The listing builds one solid part. Answer for the finished solid, in the listing's coordinates (mm). Face numbers are marked on the shaded views. A direction names the side the tool comes from. Coordinates: 2 decimals unless noted, no trailing zeros. Order: outer loops, then holes, each group sorted by start corner. A loop starts at its lowest first (then second) coordinate and runs counter-clockwise, first axis right, second up. Notation, with made-up numbers: (32, 79) - (45, 79) arc R16 ccw to (45, 84) - close; hole circle Ø5 at (19.5, 25). An arc over 180 degrees is marked (long way). Use a Markdown table: item, result. Add a question column.
Item 1: The mould has two halves that part along Y. Classify the marked faces 1, 2, 3 and 4: released by +Y, released by -Y, zero draft, split by the parting line, or undercut.
Item 2: The part is cut by section B-B, the plane x = 0. Give the vertices of the cut face in (y, z) (1 decimal), then the cut area to 3 significant figures.
Item 3: The part is cut by section A-A, the plane y = 0. Give the vertices of the cut face in (x, z) (3 decimals).
Item 4: Flat-ended cylindrical pins translate along their axes: P1, Ø10, axis at x = 0, y = 0, coming from the -Z side; P2, Ø5, axis at x = 17.78, y = 0, coming from the -Z side; P3, Ø2, axis at x = 8.5, z = 3, coming from the +Y side; P4, Ø5, axis at x = 2, z = 6.5, coming from the +Y side. Find the tip coordinate at first contact, or state that the pin passes through.
Item 5: The part is cut by section D-D, the plane x = -19.5. Give the vertices of the cut face in (y, z) (3 decimals).
Item 6: The part is cut by section C-C, the plane y = -20. Give the vertices of the cut face in (x, z) (3 decimals).
Item 7: Find the intervals of material crossed by line 1 along X through (y, z) = (-2, 6); line 2 along X through (y, z) = (-0.5, 7); line 3 along Y through (x, z) = (-2, 3.75), in increasing order.
Item 8: For the marked faces 5 and 6, determine the directions among +Z, -Z, +X, -X, +Y, -Y from which every point of the face is accessible in a straight line to the end or side of a thin tool.
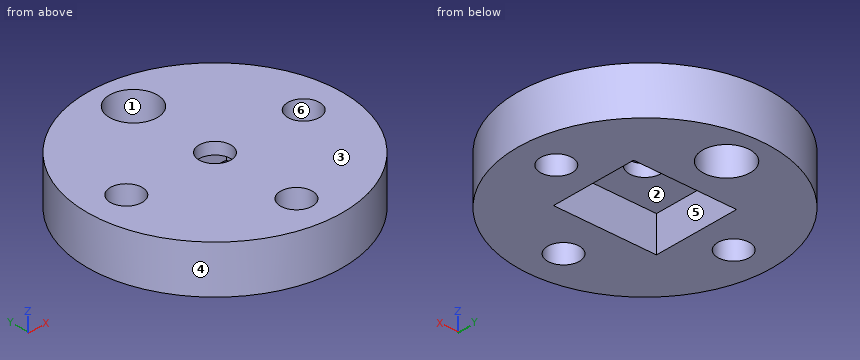
from build123d import *

# Parameters (mm, degrees)
SKETCH1_R           = 25.4
BOSS_EXTRUDE1_DEPTH = 9.525
SKETCH2_W           = 20.6375
SKETCH2_H           = 17.4625
CUT_EXTRUDE1_DEPTH  = 7.14375
SKETCH3_R           = 3.175
CUT_EXTRUDE9_DEPTH  = 15.5575
SKETCH5_R           = 4.7625
SKETCH5_R_2         = 3.175
CUT_EXTRUDE10_DEPTH = 15.5575


with BuildPart() as part:
    # Sketch1 → Boss-Extrude1 (new body)
    with BuildSketch(Plane.XY):
        with Locations(Location((0, 0, 0), (0, 0, 180))):
            Circle(SKETCH1_R)
    extrude(amount=BOSS_EXTRUDE1_DEPTH)

    # Sketch2 → Cut-Extrude1 (cut)
    with BuildSketch(Plane.XY):
        Rectangle(SKETCH2_W, SKETCH2_H)
    extrude(amount=CUT_EXTRUDE1_DEPTH, mode=Mode.SUBTRACT)

    # Sketch3 → Cut-Extrude9 (cut)
    with BuildSketch(Plane(origin=(0, 0, 7.14375), x_dir=(-1, 0, 0), z_dir=(0, 0, -1))):
        Circle(SKETCH3_R)
    extrude(amount=-CUT_EXTRUDE9_DEPTH, mode=Mode.SUBTRACT)

    # Sketch5 → Cut-Extrude10 (cut)
    with BuildSketch(Plane.XY.offset(9.525)):
        with Locations((0, 17.78)):
            Circle(SKETCH5_R)
        with Locations((17.78, 0)):
            Circle(SKETCH5_R_2)
        with Locations((0, -17.768897269)):
            Circle(SKETCH5_R_2)
        with Locations((-17.78, 0)):
            Circle(SKETCH5_R_2)
    extrude(amount=-CUT_EXTRUDE10_DEPTH, mode=Mode.SUBTRACT)


solid = part.part
Solution:
| question | item | result |
|---|---|---|
| 1 | face 1 | undercut |
| 1 | face 2 | undercut |
| 1 | face 3 | zero draft |
| 1 | face 4 | split by the parting line |
| 2 | outline | (-25.4, 0) - (-20.9, 0) - (-20.9, 9.5) - (-25.4, 9.5) - close; (-14.6, 0) - (-8.7, 0) - (-8.7, 7.1) - (-3.2, 7.1) - (-3.2, 9.5) - (-14.6, 9.5) - close; (3.2, 7.1) - (8.7, 7.1) - (8.7, 0) - (13, 0) - (13, 9.5) - (3.2, 9.5) - close; (22.5, 0) - (25.4, 0) - (25.4, 9.5) - (22.5, 9.5) - close |
| 2 | area | 193 mm2 |
| 3 | outline | (-25.4, 0) - (-20.955, 0) - (-20.955, 9.525) - (-25.4, 9.525) - close; (-14.605, 0) - (-10.319, 0) - (-10.319, 7.144) - (-3.175, 7.144) - (-3.175, 9.525) - (-14.605, 9.525) - close; (3.175, 7.144) - (10.319, 7.144) - (10.319, 0) - (14.605, 0) - (14.605, 9.525) - (3.175, 9.525) - close; (20.955, 0) - (25.4, 0) - (25.4, 9.525) - (20.955, 9.525) - close |
| 4 | P1 | stops at z = 7.14 |
| 4 | P2 | passes through |
| 4 | P3 | stops at y = 24.27 |
| 4 | P4 | stops at y = 25.4 |
| 5 | outline | (-16.276, 0) - (-2.669, 0) - (-2.669, 9.525) - (-16.276, 9.525) - close; (2.669, 0) - (16.276, 0) - (16.276, 9.525) - (2.669, 9.525) - close |
| 6 | outline | (-15.658, 0) - (-2.259, 0) - (-2.259, 9.525) - (-15.658, 9.525) - close; (2.259, 0) - (15.658, 0) - (15.658, 9.525) - (2.259, 9.525) - close |
| 7 | line 1 | x = -25.32 to -20.25, -15.31 to -10.32, 10.32 to 15.31, 20.25 to 25.32 |
| 7 | line 2 | x = -25.4 to -20.92, -14.64 to -10.32, 10.32 to 14.64, 20.92 to 25.4 |
| 7 | line 3 | y = -25.32 to -20.23, -15.3 to -8.73, 8.73 to 13.46, 22.1 to 25.32 |
| 8 | face 5 | -Z |
| 8 | face 6 | +Z, -Z |
